```python
from build123d import *

# Parameters (mm, degrees)
SKETCH2_R               = 2.6
SKETCH2_R_2             = 12.5
CUT_EXTRUDE2_DEPTH      = 75.636586376
CUT_EXTRUDE4_DEPTH      = 75.2781452
CUT_EXTRUDE4_DEPTH_BACK = 75.2781452


with BuildPart() as part:
    # Sketch1 → Revolve1 (revolve)
    with BuildSketch(Plane.XY):
        with BuildLine():
            Line((41.1, 0), (41.1, 25))
            add(Edge.make_bspline(
                [(41.1, 25), (41.1, 38), (0, 38)],
                knots=[0, 0, 0, 1.570796327, 1.570796327, 1.570796327], degree=2, weights=[1, 0.707106781, 1]))
            Line((0, 38), (0, 41))
            add(Edge.make_bspline(
                [(44.1, 25), (44.1, 41), (0, 41)],
                knots=[0, 0, 0, 1.570796327, 1.570796327, 1.570796327], degree=2, weights=[1, 0.707106781, 1]))
            Line((44.1, 25), (44.1, 0))
            Line((44.1, 0), (41.1, 0))
        make_face()
    revolve(axis=Axis((0, 38, 0), (0, 1, 0)))

    # Sketch2 → Cut-Extrude2 (cut, through all)
    with BuildSketch(Plane(origin=(0, 0, 0), x_dir=(1, 0, 0), z_dir=(0, 1, 0))):
        with Locations((25.5, 0)):
            Circle(SKETCH2_R)
        with Locations(Location((0, -25.5, 0), (0, 0, 90))):
            Circle(SKETCH2_R)
        with Locations(Location((-25.5, 0, 0), (0, 0, 90))):
            Circle(SKETCH2_R)
        with Locations(Location((0, 25.5, 0), (0, 0, 90))):
            Circle(SKETCH2_R)
        Circle(SKETCH2_R_2)
    extrude(amount=CUT_EXTRUDE2_DEPTH, mode=Mode.SUBTRACT)

    # Sketch3 → Cut-Extrude4 (cut, two sides: drawn at the far end of the back side and taken through both)
    with BuildSketch(Plane.XY.offset(-CUT_EXTRUDE4_DEPTH_BACK)):
        Polygon((0, 18.850852961), (-5.5, 15.675426481), (-5.5, 9.324573519), (0, 6.149147039), (5.5, 9.324573519), (5.5, 15.675426481), align=None)
    extrude(amount=CUT_EXTRUDE4_DEPTH + CUT_EXTRUDE4_DEPTH_BACK, mode=Mode.SUBTRACT)


solid = part.part
```
For this review, take the finished solid that the model builds, in its own axes (mm). A direction names the side the tool comes from. Round coordinates to 2 decimals unless told otherwise and drop trailing zeros. Order: outer loops, then holes, each group sorted by start corner. A loop starts at its lowest first (then second) coordinate and runs counter-clockwise, first axis right, second up.
Q1. Machinability: for faces 4 (the flat face through (-5.5, 13, -42)), 5 (the cylindrical face through (-8.91, 12.675, 40.123)), 6 (the cylindrical face through (-1.757, 36.551, 27.416)), which of the approach directions +Z, -Z, +X, -X, +Y, -Y give a long, thin tool a straight path to every point of the face, cutting with its end or side? Answer none if there is none.
Findings below:
face 4: +Z, -Z
face 5: -Y
face 6: +Y, -Y
Q2. Insertion check: P1, Ø6, axis at y = 7.5, z = 10, coming from the -X side; P2, Ø3, axis at y = 27, z = 22.5, coming from the +X side; P3, Ø8.5, axis at x = 25.5, z = 0, coming from the +Y side; P4, Ø3, axis at x = -25.5, z = 0, coming from the +Y side. Each pin has a flat end and moves straight along its axis. Give the tip position at first contact, or say it passes through.
Findings below:
P1: stops at x = -43.54
P2: stops at x = 38.52
P3: stops at y = 39.02
P4: passes through
Q3. We need section B-B, the plane z = 0. State how many separate pieces and enclosed holes the cut face has, plus the area to 3 significant figures.
Findings below:
separate pieces: 4
enclosed holes: 0
area: 315 mm2
Q4. We need section A-A, the plane y = 22. Give the boundary of the cut face in (x, z), plus the area to 3 significant figures.
Findings below:
outline: circle Ø88.2 at (0, 0); hole circle Ø82.2 at (0, 0)
area: 803 mm2
Q5. Mouldability with a two-part tool opening along X and no side actions: class faces 1 (the flat face through (-5.5, 13, 42)), 2 (the cylindrical face through (-9.56, 12.32, 43.05)), 3 (the flat face through (29.2, 0, 29.2)) as pulls with the +X half, pulls with the -X half, needs draft (parallel to the pull), parting line crosses it, or undercut.
Findings below:
face 1: undercut
face 2: parting line crosses it
face 3: needs draft
Q6. Wall thickness on line 1 (X direction, y = 2.5, z = -17); line 2 (Z direction, x = 36, y = 25); line 3 (Z direction, x = -19, y = 21): over which ranges is each line inside the solid? List them lowest first.
Findings below:
line 1: x = -40.69 to -37.42, 37.42 to 40.69
line 2: z = -25.47 to -19.83, 19.83 to 25.47
line 3: z = -39.8 to -36.44, 36.44 to 39.8
